from build123d import *

# Parameters (mm, degrees)
F0_W     = 1550.9875
F0_H     = 25.4
F1_DEPTH = 174.625
F3_W     = 1419.225
F3_H     = 25.4
F4_DEPTH = 130.175
F5_W     = 1292.225
F5_H     = 25.4
F6_DEPTH = 73.025
F2_W     = 1363.6625
F2_H     = 250.825
F7_DEPTH = 25.4
F9_DEPTH = 12.7


with BuildPart() as f1:
    # F0 (on Front) → F1 (new body)
    with BuildSketch(Plane.XZ):
        with Locations((0, -12.7)):
            Rectangle(F0_W, F0_H)
    extrude(amount=F1_DEPTH)

    # F3 (on Front) → F4 (join)
    with BuildSketch(Plane.XZ):
        with Locations((0, -38.1)):
            Rectangle(F3_W, F3_H)
    extrude(amount=F4_DEPTH)

    # F5 (on Front) → F6 (join)
    with BuildSketch(Plane.XZ):
        with Locations((0, -63.5)):
            Rectangle(F5_W, F5_H)
    extrude(amount=F6_DEPTH)

    # F2 (on Front) → F7 (join)
    with BuildSketch(Plane.XZ):
        with Locations((7.9375, -150.8125)):
            Rectangle(F2_W, F2_H)
    extrude(amount=F7_DEPTH)

    # F8 (on face) → F9 (cut)
    with BuildSketch(Plane.XZ.offset(25.4)):
        Polygon((-673.89375, -50.8), (-673.89375, -276.225), (-620.7125, -276.225), (-620.7125, -76.2), (-646.1125, -76.2), (-646.1125, -50.8), align=None)
        Polygon((620.7125, -76.2), (620.7125, -276.225), (689.76875, -276.225), (689.76875, -50.8), (646.1125, -50.8), (646.1125, -76.2), align=None)
    extrude(amount=-F9_DEPTH, mode=Mode.SUBTRACT)


solid = f1.part
Verification items for the finished model (mm, model axes). A direction names the side the tool comes from. Give positions to 0.01 mm unless a question says otherwise; leave off trailing zeros. Loops run counter-clockwise (first coordinate to the right, second up) from the corner with the lowest first, then second, coordinate; pieces in that order, holes last.
1) Sectioned sample at C-C, the plane x = -580. Enter the section's corners in (y, z) (3 decimals), then the cut area to 3 significant figures.
2) Depth check by flat-ended pin: pin 1 Ø6.5 at (y, z) = (-19.5, -187) entering from +X; pin 2 Ø7.5 at (y, z) = (-56, -65.5) entering from -X; pin 3 Ø12 at (x, z) = (293, -95) entering from -Y. Enter the tip coordinate at first touch or a pass-through.
3) Set-up check for faces 1 (the flat face through (-646.112, -42, -64)), 2 (the flat face through (-709.612, -64, -38)), 3 (the flat face through (-9, -25.4, -175)): record each of +Z, -Z, +X, -X, +Y, -Y from which the full face is reachable in a straight line by a thin tool's end or side.
4) Thickness scan on line 1 along Y through (x, z) = (-290, -145.5); line 2 along Z through (x, y) = (703.5, -72.5); line 3 along Z through (x, y) = (-348.5, -41). Record the ranges inside material, lowest first.
5) Sectioned sample at A-A, the plane z = -116.5. Enter the section's corners in (x, y), then the cut area to 3 significant figures.
6) Sectioned sample at B-B, the plane y = -49. Enter the section's corners in (x, z), then the cut area to 3 significant figures.
Answers:
1. outline: (-174.625, -25.4) - (-130.175, -25.4) - (-130.175, -50.8) - (-73.025, -50.8) - (-73.025, -76.2) - (-25.4, -76.2) - (-25.4, -276.225) - (0, -276.225) - (0, 0) - (-174.625, 0) - close
1. area: 14,700 mm2
2. pin 1: stops at x = 620.71
2. pin 2: stops at x = -646.11
2. pin 3: stops at y = -25.4
3. face 1: -Z, -X, -Y
3. face 2: -Z, -X, +Y, -Y
3. face 3: -Z, +X, -X, -Y
4. line 1: y = -25.4 to 0
4. line 2: z = -50.8 to 0
4. line 3: z = -76.2 to 0
5. outline: (-673.89, -12.7) - (-620.71, -12.7) - (-620.71, -25.4) - (620.71, -25.4) - (620.71, -12.7) - (689.77, -12.7) - (689.77, 0) - (-673.89, 0) - close
5. area: 33,100 mm2
6. outline: (-775.49, -25.4) - (-709.61, -25.4) - (-709.61, -50.8) - (-646.11, -50.8) - (-646.11, -76.2) - (646.11, -76.2) - (646.11, -50.8) - (709.61, -50.8) - (709.61, -25.4) - (775.49, -25.4) - (775.49, 0) - (-775.49, 0) - close
6. area: 108,000 mm2
